from build123d import *

# Parameters (mm, degrees)
SKETCH_2_R          = 11.5
CUT_EXTRUDE_1_DEPTH = 312.628785577


with BuildPart() as part:
    # Эскиз1 → Повернуть1 (revolve)
    with BuildSketch(Plane.XY, mode=Mode.PRIVATE) as revolve_1_sk:
        with BuildLine():
            Line((-150, 0), (-150, 50))
            Line((-150, 50), (-178.5, 50))
            Line((-178.5, 50), (-178.5, 54))
            Line((-178.5, 54), (-182.5, 54))
            Line((-182.5, 54), (-183.5, 50))
            Line((-183.5, 50), (-217.5, 50))
            Line((-217.5, 50), (-217.5, 34))
            ThreePointArc((-217.5, 34), (-216.914213562, 32.585786438), (-215.5, 32))
            Line((-215.5, 32), (-175.991183949, 32))
            ThreePointArc((-175.991183949, 32), (-171.439506628, 30.318104321), (-169.075099713, 26.080638162))
            Line((-169.075099713, 26.080638162), (-165, 0))
            Line((-165, 0), (-150, 0))
        make_face()
    revolve(revolve_1_sk.sketch.rotate(Axis((0, 0, 0), (0, 1, 0)), 270), axis=Axis((0, 0, 0), (0, 1, 0)))

    # Эскиз2 → Вырез-Вытянуть1 (cut, through all)
    with BuildSketch(Plane(origin=(0, 50, 0), x_dir=(1, 0, 0), z_dir=(0, 1, 0))):
        with Locations(Location((-197.5, 0, 0), (0, 0, 270))):
            Circle(SKETCH_2_R)
        with Locations(Location((-171.040017247, 98.75, 0), (0, 0, 270))):
            Circle(SKETCH_2_R)
        with Locations(Location((-98.75, 171.040017247, 0), (0, 0, 270))):
            Circle(SKETCH_2_R)
        with Locations(Location((0, 197.5, 0), (0, 0, 270))):
            Circle(SKETCH_2_R)
        with Locations(Location((98.75, 171.040017247, 0), (0, 0, 270))):
            Circle(SKETCH_2_R)
        with Locations(Location((171.040017247, 98.75, 0), (0, 0, 270))):
            Circle(SKETCH_2_R)
        with Locations(Location((197.5, 0, 0), (0, 0, 270))):
            Circle(SKETCH_2_R)
        with Locations(Location((171.040017247, -98.75, 0), (0, 0, 270))):
            Circle(SKETCH_2_R)
        with Locations(Location((98.75, -171.040017247, 0), (0, 0, 270))):
            Circle(SKETCH_2_R)
        with Locations(Location((0, -197.5, 0), (0, 0, 270))):
            Circle(SKETCH_2_R)
        with Locations(Location((-98.75, -171.040017247, 0), (0, 0, 270))):
            Circle(SKETCH_2_R)
        with Locations(Location((-171.040017247, -98.75, 0), (0, 0, 270))):
            Circle(SKETCH_2_R)
    extrude(amount=-CUT_EXTRUDE_1_DEPTH, mode=Mode.SUBTRACT)


solid = part.part
Geometry check sheet. Reference: the model listing, model coordinates, mm. A direction names the side the tool comes from. Coordinates: 2 decimals unless noted, no trailing zeros. Answer in a Markdown table with one row per item. Add a question column.
1) Set-up check for faces 1 (the cylindrical face through (174.255, 52.028, 38.695)), 2 (the flat face through (175, 32, -31)), 3 (the cylindrical face through (0.51, 41.13, 186.01)): record each of +Z, -Z, +X, -X, +Y, -Y from which the full face is reachable in a straight line by a thin tool's end or side.
2) Release check for a two-part mould opening along X. For faces 4 (the flat face through (-130, 50, -130)), 5 (the cylindrical face through (-105.748, 41.126, 161.914)), 6 (the conical face through (-49.62, 1.27, -157.57)) record: +X half, -X half, draft (parallel to the pull), parting line (faces both ways), or undercut.
3) Gauge pin test, flat ends, axial feed: P1, Ø5, axis at y = 34, z = 120, coming from the +X side; P2, Ø20.5, axis at x = -98.75, z = 171.04, coming from the -Y side; P3, Ø8, axis at y = 20.5, z = 83.5, coming from the -X side; P4, Ø1, axis at y = 17.5, z = 26.5, coming from the +X side. Record the tip position at first contact, or that the pin passes through.
4) Cross-section at A-A, the plane x = 0. State how many separate pieces and enclosed holes the cut face has, then the cut area to 3 significant figures.
5) Material ranges on line 1 along Z through (x, y) = (107, 41.5); line 2 along X through (y, z) = (45.5, -98.75); line 3 along Z through (x, y) = (-164.5, 37.5), recorded low to high. Write a range as [from, to].
Check result:
| question | item | result |
|---|---|---|
| 1 | face 1 | +Y |
| 1 | face 2 | -Y |
| 1 | face 3 | +Y, -Y |
| 2 | face 4 | draft |
| 2 | face 5 | undercut |
| 2 | face 6 | parting line |
| 3 | P1 | stops at x = 183.03 |
| 3 | P2 | passes through |
| 3 | P3 | stops at x = -148.34 |
| 3 | P4 | stops at x = 165.74 |
| 4 | separate pieces | 4 |
| 4 | enclosed holes | 0 |
| 4 | area | 2,770 mm² |
| 5 | line 1 | z = [-189.36, -179.05], [-163.03, -105.12], [105.12, 163.03], [179.05, 189.36] |
| 5 | line 2 | x = [-193.79, -182.54], [-159.54, -112.91], [112.91, 159.54], [182.54, 193.79] |
| 5 | line 3 | z = [-142.29, -108.21], [-89.29, 89.29], [108.21, 142.29] |
